```python
from build123d import *
from OCP.BRepFilletAPI import BRepFilletAPI_MakeChamfer

# Parameters (mm, degrees)
BOSS_EXTRU_1_DEPTH      = 15
CHANFREIN1_SIZE         = 10.503113073
CHANFREIN1_SIZE_2       = 15
ESQUISSE4_R             = 2
ENL_V_MAT_EXTRU_3_DEPTH = 4
ENL_V_MAT_EXTRU_5_DEPTH = 5
ESQUISSE6_R             = 2
ENL_V_MAT_EXTRU_6_DEPTH = 5


with BuildPart() as part:
    # Esquisse1 → Boss.-Extru.1 (new body)
    with BuildSketch(Plane(origin=(0, 0, 0), x_dir=(1, 0, 0), z_dir=(0, 1, 0))):
        Polygon((-41.352348911, -18.647651089), (8.647651089, -18.647651089), (8.647651089, -68.647651089), (68.647651089, -68.647651089), (117.647651089, -68.647651089), (117.647651089, -46.647651089), (68.647651089, -46.647651089), (30.647651089, -46.647651089), (30.647651089, 3.352348911), (-19.352348911, 3.352348911), (-19.352348911, 41.352348911), (-41.352348911, 41.352348911), align=None)
    extrude(amount=BOSS_EXTRU_1_DEPTH)

    # Chanfrein1
    chanfrein1_edges_1 = [part.edges().sort_by_distance(p)[0] for p in [
        (63.147651089, 15, 68.647651089),
    ]]
    chanfrein1_side_1 = [part.faces().sort_by_distance(p)[0] for p in [
        (63.147651089, 15, 68.437588827),
    ]]
    chanfrein1_edges_2 = [part.edges().sort_by_distance(p)[0] for p in [
        (8.647651089, 15, 43.647651089),
    ]]
    chanfrein1_side_2 = [part.faces().sort_by_distance(p)[0] for p in [
        (8.85771335, 15, 43.647651089),
    ]]
    chanfrein1_edges_3 = [part.edges().sort_by_distance(p)[0] for p in [
        (-16.352348911, 15, 18.647651089),
    ]]
    chanfrein1_side_3 = [part.faces().sort_by_distance(p)[0] for p in [
        (-16.352348911, 14.789937739, 18.647651089),
    ]]
    chanfrein1_edges_4 = [part.edges().sort_by_distance(p)[0] for p in [
        (-41.352348911, 15, -11.352348911),
    ]]
    chanfrein1_side_4 = [part.faces().sort_by_distance(p)[0] for p in [
        (-41.14228665, 15, -11.352348911),
    ]]
    chanfrein1 = BRepFilletAPI_MakeChamfer(part.part.solid().wrapped)
    for e in chanfrein1_edges_1:
        chanfrein1.Add(CHANFREIN1_SIZE - 0.0001, CHANFREIN1_SIZE_2 - 0.0001, e.wrapped, chanfrein1_side_1[0].wrapped)
    for e in chanfrein1_edges_2:
        chanfrein1.Add(CHANFREIN1_SIZE - 0.0001, CHANFREIN1_SIZE_2 - 0.0001, e.wrapped, chanfrein1_side_2[0].wrapped)
    for e in chanfrein1_edges_3:
        chanfrein1.Add(CHANFREIN1_SIZE_2 - 0.0001, CHANFREIN1_SIZE - 0.0001, e.wrapped, chanfrein1_side_3[0].wrapped)
    for e in chanfrein1_edges_4:
        chanfrein1.Add(CHANFREIN1_SIZE - 0.0001, CHANFREIN1_SIZE_2 - 0.0001, e.wrapped, chanfrein1_side_4[0].wrapped)
    add(Compound.cast(chanfrein1.Shape()), mode=Mode.REPLACE)  # a hair under: the kernel refuses the full size

    # Esquisse4 → Enlèv. mat.-Extru.3 (cut)
    with BuildSketch(Plane.XZ):
        with Locations(Location((38.647651089, 63.647651089, 0), (0, 0, 270))):
            Circle(ESQUISSE4_R)
        with Locations(Location((13.647651089, 38.647651089, 0), (0, 0, 270))):
            Circle(ESQUISSE4_R)
        with Locations(Location((-11.352348911, 13.647651089, 0), (0, 0, 270))):
            Circle(ESQUISSE4_R)
    extrude(amount=-ENL_V_MAT_EXTRU_3_DEPTH, mode=Mode.SUBTRACT)

    # Esquisse5 → Enlèv. mat.-Extru.5 (cut)
    with BuildSketch(Plane(origin=(0, 15, 0), x_dir=(1, 0, 0), z_dir=(0, 1, 0))):
        Polygon((-28.849235838, 41.352348911), (-19.352348911, 41.352348911), (-19.352348911, 3.352348911), (30.647651089, 3.352348911), (30.647651089, -46.647651089), (117.647651089, -46.647651089), (117.647651089, -56.140382231), (21.150764162, -56.140382231), (21.150764162, -6.144538016), (-28.849235838, -6.144538016), align=None)
    extrude(amount=-ENL_V_MAT_EXTRU_5_DEPTH, mode=Mode.SUBTRACT)

    # Esquisse6 → Enlèv. mat.-Extru.6 (cut)
    with BuildSketch(Plane(origin=(0, 10, 0), x_dir=(1, 0, 0), z_dir=(0, 1, 0))):
        with Locations(Location((-23.849235838, 28.855461984, 0), (0, 0, 270))):
            Circle(ESQUISSE6_R)
        with Locations(Location((26.150764162, -1.144538016, 0), (0, 0, 270))):
            Circle(ESQUISSE6_R)
        with Locations(Location((106.150456792, -50.918618661, 0), (0, 0, 270))):
            Circle(ESQUISSE6_R)
    extrude(amount=-ENL_V_MAT_EXTRU_6_DEPTH, mode=Mode.SUBTRACT)


solid = part.part
```
Build history of the part. All positions in model axes, mm. A direction names the side the tool comes from. Give positions to 0.01 mm unless a question says otherwise; leave off trailing zeros. Loops run counter-clockwise (first coordinate to the right, second up) from the corner with the lowest first, then second, coordinate; pieces in that order, holes last.
1) Probe line 1 along Y through (x, z) = (30, 34); line 2 along Y through (x, z) = (25, 0); line 3 along X through (y, z) = (8, 1.5). List the from-to ranges inside material, lowest first.
Values follow:
line 1: y = 0 to 10
line 2: y = 0 to 5
line 3: x = -35.75 to 24.18, 28.12 to 30.65
2) Two-plate mould, pull along Z, no slides. Class faces 1 (the face through (28, 10, 25)), 2 (the face through (75, 5, 46.648)), 3 (the face through (-21.866, 7.535, -29.116)): released by +Z, released by -Z, zero draft, split by the parting line, or undercut.
Values follow:
face 1: zero draft
face 2: released by -Z
face 3: undercut
3) 3-axis set-ups, long thin cutter, end or side, ignore diameter. For faces 4 (the face through (13.83, 7.4, 37.97)), 5 (the face through (70, 13, 56.14)), 6 (the face through (11.7, 2, 39.1)): which of +Z, -Z, +X, -X, +Y, -Y reach the whole face in a straight line?
Values follow:
face 4: +Z, -X, +Y
face 5: -Z, +X, +Y
face 6: -Y
4) Drop flat-ended pins along their axis: P1, Ø5, axis at x = 11, y = 3, coming from the -Z side; P2, Ø4, axis at x = 65.5, y = 11.5, coming from the -Z side; P3, Ø1.5, axis at y = 2, z = -18.5, coming from the +X side. Give the stop position or say it passes through.
Values follow:
P1: stops at z = -3.35
P2: stops at z = 46.65
P3: stops at x = -19.35
5) Band-saw the part on B-B on y = 7.5. List the corners of the cut face in (x, z).
Values follow:
outline: (-36.1, -41.35) - (-19.35, -41.35) - (-19.35, -3.35) - (30.65, -3.35) - (30.65, 46.65) - (117.65, 46.65) - (117.65, 63.4) - (13.9, 63.4) - (13.9, 13.4) - (-36.1, 13.4) - close; hole circle Ø4 at (-23.85, -28.86); hole circle Ø4 at (26.15, 1.14); hole circle Ø4 at (106.15, 50.92)
